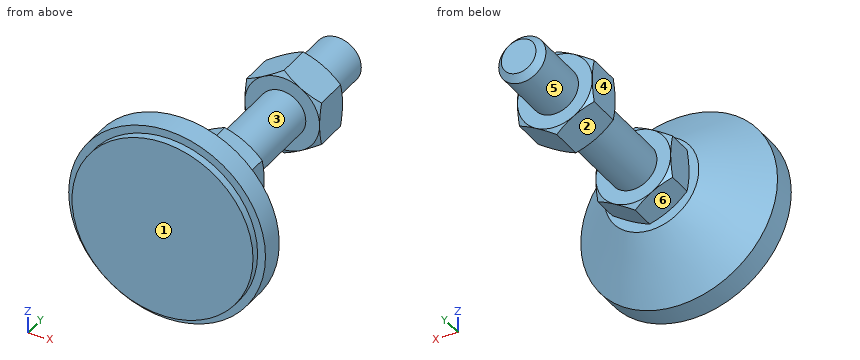
```python
from build123d import *

# Parameters (mm, degrees)
EXTRUDE_1_DEPTH = 8
EXTRUDE_2_DEPTH = 10


with BuildPart() as part:
    # Эскиз1 → Повернуть1 (revolve)
    with BuildSketch(Plane.XY, mode=Mode.PRIVATE) as revolve_1_sk:
        Polygon((0, 0), (-23, 0), (-23, 2), (-25, 2), (-25, 8), (-12, 20), (-6, 20), (-6, 28), (-6, 76.4), (-4.4, 78), (0, 78), align=None)
    revolve(revolve_1_sk.sketch.rotate(Axis((0, 0, 0), (0, 1, 0)), 180), axis=Axis((0, 0, 0), (0, 1, 0)))  # turned: the seam where the file's is

    # Эскиз2 → Бобышка-Вытянуть1 (add)
    with BuildSketch(Plane(origin=(0, 20, 0), x_dir=(1, 0, 0), z_dir=(0, 1, 0))):
        Polygon((0, 10.969655115), (-9.5, 5.484827557), (-9.5, -5.484827557), (0, -10.969655115), (9.5, -5.484827557), (9.5, 5.484827557), align=None)
    extrude(amount=EXTRUDE_1_DEPTH)

    # Эскиз3 → Бобышка-Вытянуть2 (add)
    with BuildSketch(Plane(origin=(0, 52.2, 0), x_dir=(1, 0, 0), z_dir=(0, 1, 0))):
        Polygon((9.5, 5.484827557), (0, 10.969655115), (-9.5, 5.484827557), (-9.5, -5.484827557), (0, -10.969655115), (9.5, -5.484827557), align=None)
    extrude(amount=EXTRUDE_2_DEPTH)

    # Эскиз4 → Вырез-Повернуть2 (revolve, cut)
    with BuildSketch(Plane.XY, mode=Mode.PRIVATE) as cut_revolve_2_sk:
        Polygon((-18.160254038, 62.2), (-9.5, 62.2), (-18.160254038, 57.2), align=None)
        Polygon((-18.160254038, 52.2), (-18.160254038, 57.2), (-9.5, 52.2), align=None)
        Polygon((-16.42820323, 28), (-16.42820323, 24), (-9.5, 28), align=None)
        Polygon((-16.42820323, 24), (-16.42820323, 20), (-9.5, 20), align=None)
    revolve(cut_revolve_2_sk.sketch.rotate(Axis((0, 78, 0), (0, 1, 0)), 180), axis=Axis((0, 78, 0), (0, 1, 0)), mode=Mode.SUBTRACT)  # turned: the seam where the file's is


solid = part.part
```
Design review of the part built by this model. Coordinates are the model's own, in mm. Face numbers are marked on the shaded views. A direction names the side the tool comes from. Coordinates: 2 decimals unless noted, no trailing zeros. Order: outer loops, then holes, each group sorted by start corner. A loop starts at its lowest first (then second) coordinate and runs counter-clockwise, first axis right, second up.
1) Take a section at A-A, the plane y = 56. Give the boundary of the cut face in (x, z), and give its area (3 significant figures).
2) Mouldability with a two-part tool opening along Y and no side actions: class the marked faces 1, 2 and 3 as +Y half, -Y half, draft (parallel to the pull), parting line (faces both ways), or undercut.
3) For the marked faces 4, 5 and 6, list the 3-axis set-ups (+Z, -Z, +X, -X, +Y, -Y) from which the entire face can be reached by the end or side of a thin tool; tool diameter is ignored.
4) Take a section at B-B, the plane y = 6.5. Give the boundary of the cut face in (x, z).
5) Clearance check with flat-ended pins moving along their axes: pin 1 (6 mm diameter, centred on y = 39, z = -1.5, fed in from +X); pin 2 (1.5 mm diameter, centred on x = -3.5, y = 61, fed in from +Z); pin 3 (2.5 mm diameter, centred on y = 23.5, z = 1, fed in from -X). State where each tip first meets the part, or that it passes through.
6) Wall thickness on line 1 along Z through (x, y) = (0, 73.5); line 2 along Z through (x, y) = (-3.5, 64); line 3 along Y through (x, z) = (-8, -9.5): over which ranges is each line inside the solid? List them lowest first.
Returned:
1. outline: (-9.5, -5.48) - (0, -10.97) - (9.5, -5.48) - (9.5, 5.48) - (0, 10.97) - (-9.5, 5.48) - close
1. area: 313 mm2
2. face 1: -Y half
2. face 2: draft
2. face 3: undercut
3. face 4: +Z, -Z, -X, +Y
3. face 5: +Y
3. face 6: -Z, -X, +Y
4. outline: circle Ø50 at (0, 0)
5. pin 1: stops at x = 6
5. pin 2: stops at z = 9.38
5. pin 3: stops at x = -9.5
6. line 1: z = -6 to 6
6. line 2: z = -4.87 to 4.87
6. line 3: y = 0 to 19.61
